```python
from build123d import *

# Parameters (mm, degrees)
ESQUISSE1_W             = 80
ESQUISSE1_H             = 80
BOSS_EXTRU_1_DEPTH      = 25.25
ENL_V_MAT_EXTRU_1_DEPTH = 25.25


with BuildPart() as part:
    # Esquisse1 → Boss.-Extru.1 (new body)
    with BuildSketch(Plane.XY):
        with Locations((40, 40)):
            Rectangle(ESQUISSE1_W, ESQUISSE1_H)
    extrude(amount=BOSS_EXTRU_1_DEPTH)

    # Esquisse2 → Enlèv. mat.-Extru.1 (cut)
    with BuildSketch(Plane.XY.offset(25.25)):
        Polygon((11.787944312, 63.60583742), (25.026815154, 33.864532302), (47.069224154, 43.676361494), align=None)
        Polygon((34.444148003, 21.326107713), (56.460422486, 33.864532302), (70.917940935, 8.478512531), align=None)
    extrude(amount=-ENL_V_MAT_EXTRU_1_DEPTH, mode=Mode.SUBTRACT)


solid = part.part
```
Can you work these out from the model? Positions are in its coordinate system, mm. A direction names the side the tool comes from. Give positions to 0.01 mm unless a question says otherwise; leave off trailing zeros. Order: outer loops, then holes, each group sorted by start corner. A loop starts at its lowest first (then second) coordinate and runs counter-clockwise, first axis right, second up. Notation, with made-up numbers: M -6.75,69.25 L 0.25,69.25 A9 cw 0.25,73.25 Z; hole C 35,33.25 d7. An arc over 180 degrees is marked long. Write item = value, one per line. Start each with the question number.
Q1. Suppose I cut it at C-C (y = 60.5). Write out the boundary of the cut face in (x, z), plus the area to 3 significant figures.
Q2. For faces 1 (the flat face through (29.68, 53.5, 12.8)), 2 (the flat face through (39, 80, 12)), which set-ups out of +Z, -Z, +X, -X, +Y, -Y let a thin tool reach every point of the face, with its end or its side?
Q3. Suppose I cut it at D-D (x = 60). Write out the boundary of the cut face in (y, z), plus the area to 3 significant figures.
Q4. I need wall thicknesses on probe 1 along Y at (x, z) = (42.5, 18); probe 2 along X at (y, z) = (42.5, 14.25); probe 3 along Y at (x, z) = (64, 15). Which ranges of each line are inside material? Lowest first, please. Write a range as [from, to].
Q5. Suppose I cut it at B-B (x = 42.5). Write out the boundary of the cut face in (y, z), plus the area to 3 significant figures.
Q6. Suppose I cut it at A-A (z = 16.5). Write out the boundary of the cut face in (x, y).
Q7. We'd pull the mould along X, two halves only. Please class faces 3 (the flat face through (39, 49, 25.25)), 4 (the flat face through (45.3, 27.51, 12.8)), 5 (the flat face through (63.588, 21.349, 12.802)), 6 (the flat face through (80, 39, 12)): pulls with the +X half, pulls with the -X half, needs draft (parallel to the pull), parting line crosses it, or undercut.
Check result:
q1.outline = M 0,0 L 13.17,0 L 13.17,25.25 L 0,25.25 Z; M 17.29,0 L 80,0 L 80,25.25 L 17.29,25.25 Z
q1.area = 1,920 mm2
q2.face_1 = +Z, -Z
q2.face_2 = +Z, -Z, +X, -X, +Y
q3.outline = M 0,0 L 12.32,0 L 12.32,25.25 L 0,25.25 Z; M 27.65,0 L 80,0 L 80,25.25 L 27.65,25.25 Z
q3.area = 1,630 mm2
q4.probe_1 = [0, 18.49], [25.91, 41.64], [46.26, 80]
q4.probe_2 = [0, 21.18], [44.43, 80]
q4.probe_3 = [0, 10.92], [20.63, 80]
q5.outline = M 0,0 L 18.49,0 L 18.49,25.25 L 0,25.25 Z; M 25.91,0 L 41.64,0 L 41.64,25.25 L 25.91,25.25 Z; M 46.26,0 L 80,0 L 80,25.25 L 46.26,25.25 Z
q5.area = 1,720 mm2
q6.outline = M 0,0 L 80,0 L 80,80 L 0,80 Z; hole M 11.79,63.61 L 25.03,33.86 L 47.07,43.68 Z; hole M 34.44,21.33 L 70.92,8.48 L 56.46,33.86 Z
q7.face_3 = needs draft
q7.face_4 = undercut
q7.face_5 = undercut
q7.face_6 = pulls with the +X half
